Verification items for the finished model (mm, model axes). A direction names the side the tool comes from. Round coordinates to 2 decimals unless told otherwise and drop trailing zeros. Write each loop counter-clockwise with the first axis right and the second up, starting at its lowest first coordinate (ties: lowest second). Pieces come first, ordered by that corner, then holes. Notation, with made-up numbers: M 15,-24.5 L 44,-24.5 A19 ccw 44,10.5 Z; hole C -10.75,46.5 d4. An arc over 180 degrees is marked long. One line per question, with ' | ' between items. Start each with the question number.
Q1. Cross-section at B-B (z = -4). Record the boundary of the cut face in (x, y).
Q2. Cross-section at A-A (z = 16). Record the boundary of the cut face in (x, y).
Q3. Release check for a two-part mould opening along X. For faces 1 (the face through (1.267, -2.155, -0.28)), 2 (the face through (0.748, 0.976, 15.538)), 3 (the face through (1, -1, 20)) record: released by +X, released by -X, zero draft, split by the parting line, or undercut.
Q4. Tool access check on faces 4 (the face through (-1.15, -1.24, -20)), 5 (the face through (0, 0, -26)). Record the directions out of +Z, -Z, +X, -X, +Y, -Y that give a thin tool (end or side, any length) a straight path to the whole face; none if there is none.
Q5. Cross-section at D-D (y = -2.2). Record the boundary of the cut face in (x, z), then the cut area to 3 significant figures.
Q6. Gauge pin test, flat end, axial feed: pin 1 (2 mm diameter, centred on x = -1.5, z = -9.5, fed in from -Y). Record the tip position at first contact, or that the pin passes through.
Q7. Thickness scan on line 1 along X through (y, z) = (0, 13.5); line 2 along Y through (x, z) = (0, 17.25); line 3 along Z through (x, y) = (1.3, -1.65). Record the ranges inside material, lowest first. Write a range as from..to.
Q8. Cross-section at C-C (x = -2.1). Record the boundary of the cut face in (y, z), then the cut area to 3 significant figures.
Autodesk Inventor part; units mm, degrees
ref_plane "YZ Plane" through (0, 0, 0) normal (1, 0, 0) x (0, 1, 0)
ref_plane "XZ Plane" through (0, 0, 0) normal (0, 1, 0) x (-1, 0, 0)
ref_plane "XY Plane" through (0, 0, 0) normal (0, 0, 1) x (1, 0, 0)
sketch "Skizze1" plane through (0, 0, 0) normal (0, 0, 1) x (1, 0, 0)
  line L0 (-2.5, 1.4434) -> (0, 2.8868)
  line L1 (0, 2.8868) -> (2.5, 1.4434)
  line L2 (2.5, 1.4434) -> (2.5, -1.4434)
  line L3 (2.5, -1.4434) -> (0, -2.8868)
  line L4 (0, -2.8868) -> (-2.5, -1.4434)
  line L5 (-2.5, -1.4434) -> (-2.5, 1.4434)
  point P0 (0, 0)
  point P1 (0, 0)
  point P2 (0, 0)
  dimension "d2" = 5
extrude "Extrusion1" add sketch "Skizze1" along normal mid plane 40
sketch "Skizze3" plane through (0, 0, 20) normal (0, 0, 1) x (1, 0, 0)
  point P0 (0, 0)
  point P1 (0, 0)
hole "Bohrung1" at (0, 0, 20) direction (0, 0, -1) diameter 2.459 depth 8.8 tip angle 118
sketch "Skizze4" plane through (0, 0, -20) normal (0, 0, -1) x (-1, 0, 0)
  circle A0 centre (0, 0) radius 1.5
  dimension "d17" = 3
extrude "Extrusion3" add sketch "Skizze4" along normal blind 6
thread "Gewinde2"
chamfer "Fase1" distance 0.25 angle 45 1 edges at (1.5, 0, -26)
properties part number "standoff (1466814)"
Determined:
1) outline: M -2.5,-1.44 L 0,-2.89 L 2.5,-1.44 L 2.5,1.44 L 0,2.89 L -2.5,1.44 Z
2) outline: M -2.5,-1.44 L 0,-2.89 L 2.5,-1.44 L 2.5,1.44 L 0,2.89 L -2.5,1.44 Z; hole C 0,0 d2.46
3) face 1: released by +X | face 2: undercut | face 3: zero draft
4) face 4: -Z | face 5: -Z, +X, -X, +Y, -Y
5) outline: M -1.19,-20 L 1.19,-20 L 1.19,20 L -1.19,20 Z | area: 95.2 mm²
6) pin 1: stops at y = -2.6
7) line 1: x = -2.5..-1.23, 1.23..2.5 | line 2: y = -2.89..-1.23, 1.23..2.89 | line 3: z = -20..20
8) outline: M -1.67,-20 L 1.67,-20 L 1.67,20 L -1.67,20 Z | area: 134 mm²
